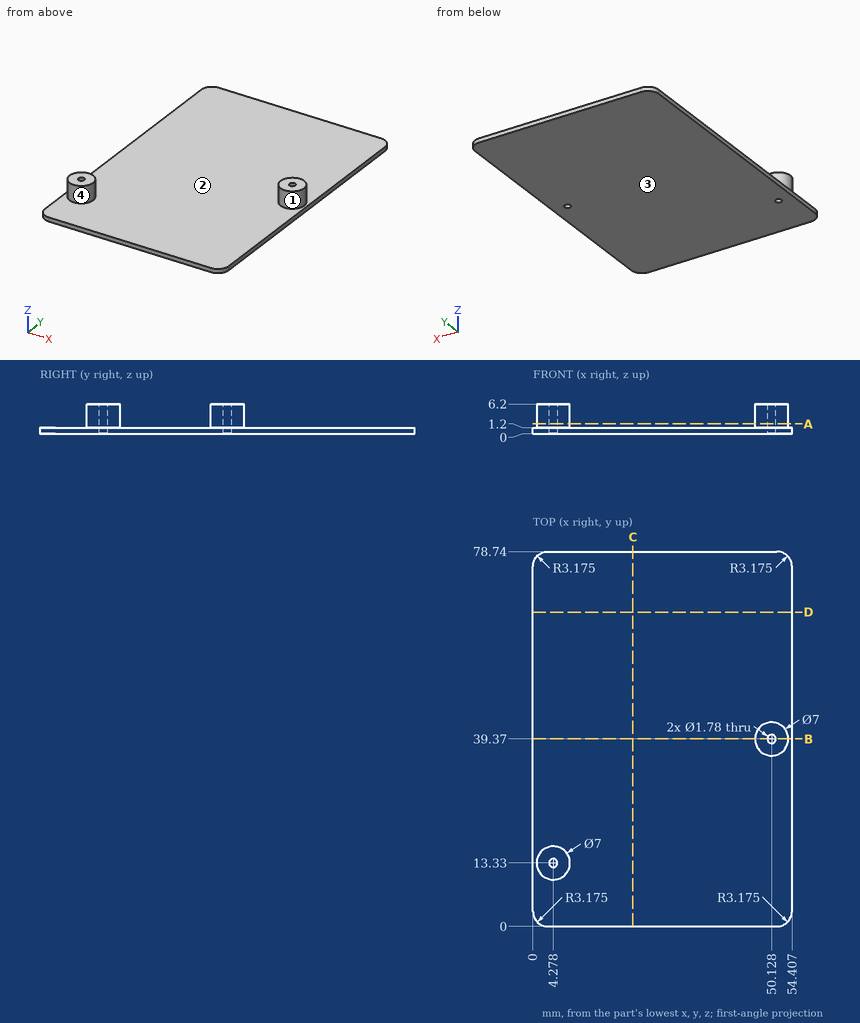
Geometry check sheet. Reference: drawing and pictorial views, mm from the part's lowest x, y, z. A direction names the side the tool comes from. Give positions to 0.01 mm unless a question says otherwise; leave off trailing zeros. Write each loop counter-clockwise with the first axis right and the second up, starting at its lowest first coordinate (ties: lowest second). Pieces come first, ordered by that corner, then holes. Notation, with made-up numbers: M 83.5,8.25 L 111.5,8.25 A32 cw 111.5,39.25 Z; hole C -13,-8.75 d3. An arc over 180 degrees is marked long. Put each result on its own line as item: value. Start each with the question number.
1. Go/stop test with a flat-tipped pin: pin 1 Ø4 at (x, y) = (48.5, 15.5) entering from +Z. Record where the tip stops, or that it passes through.
2. Section check C-C (x = 21). Record the cut outline in (y, z).
3. Draft check along X on the marked faces 1 and 2. Enter one of: +X half, -X half, draft (parallel to the pull), parting line (faces both ways), or undercut.
4. Section check B-B (y = 39.37). Record the cut outline in (x, z).
5. Section check A-A (z = 2). Record the cut outline in (x, y).
6. Set-up check for the marked faces 3 and 4: record each of +Z, -Z, +X, -X, +Y, -Y from which the full face is reachable in a straight line by a thin tool's end or side.
7. Section check D-D (y = 66). Record the cut outline in (x, z).
8. Scan lines: line 1 along X through (y, z) = (13.33, 2.5); line 2 along Z through (x, y) = (33, 44); line 3 along X through (y, z) = (13, 6) (1 decimal). Record each from-to range of solid material in increasing order. Write a range as [from, to].
Answer list:
1. pin 1: z = 1.2
2. outline: M 0,0 L 78.74,0 L 78.74,1.2 L 0,1.2 Z
3. face 1: parting line
3. face 2: draft
4. outline: M 0,0 L 49.24,0 L 49.24,6.2 L 46.63,6.2 L 46.63,1.2 L 0,1.2 Z; M 51.02,0 L 54.41,0 L 54.41,1.2 L 53.63,1.2 L 53.63,6.2 L 51.02,6.2 Z
5. outline: C 4.28,13.33 d7; C 50.13,39.37 d7; hole C 4.28,13.33 d1.78; hole C 50.13,39.37 d1.78
6. face 3: -Z, +X, -X, +Y, -Y
6. face 4: +Z
7. outline: M 0,0 L 54.41,0 L 54.41,1.2 L 0,1.2 Z
8. line 1: [0.78, 3.39], [5.17, 7.78]
8. line 2: [0, 1.2]
8. line 3: [0.8, 3.5], [5.1, 7.8]
